Here's how the part is built. I have some questions about the finished solid (model axes, mm). A direction names the side the tool comes from. Round coordinates to 2 decimals unless told otherwise and drop trailing zeros. Order: outer loops, then holes, each group sorted by start corner. A loop starts at its lowest first (then second) coordinate and runs counter-clockwise, first axis right, second up. Notation, with made-up numbers: (-11, 47) - (31, 47) arc R24 cw to (31, 69) - close; hole circle Ø10 at (24, -27.5). An arc over 180 degrees is marked (long way). One line per item, written item: value.
from build123d import *

# Parameters (mm, degrees)
BOSS_EXTRUDE1_DEPTH = 60
FILLET2_R           = 5
SKETCH5_R           = 5.5
CUT_EXTRUDE1_DEPTH  = 105.256230261


with BuildPart() as part:
    # Sketch2 → Boss-Extrude1 (new body)
    with BuildSketch(Plane.XY):
        with BuildLine():
            Line((-26, 45.665759035), (-26, 5.665759035))
            ThreePointArc((-26, 5.665759035), (0, -15.794380862), (26, 5.665759035))
            Line((26, 5.665759035), (26, 45.665759035))
            Line((26, 45.665759035), (36, 45.665759035))
            Line((36, 45.665759035), (36, 2.642754473))
            Line((36, 2.642754473), (36, -34.334240965))
            Line((36, -34.334240965), (-36, -34.334240965))
            Line((-36, -34.334240965), (-36, 5.665759035))
            Line((-36, 5.665759035), (-36, 45.665759035))
            Line((-36, 45.665759035), (-26, 45.665759035))
        make_face()
    extrude(amount=BOSS_EXTRUDE1_DEPTH)

    # Fillet2
    fillet2_edges = [part.edges().sort_by_distance(p)[0] for p in [
        (36, 45.665759035, 30),
        (26, 45.665759035, 30),
        (-26, 45.665759035, 30),
        (-36, 45.665759035, 30),
    ]]
    fillet(fillet2_edges, radius=FILLET2_R - 0.0001)  # a hair under: the kernel refuses the full size

    # Sketch5 → Cut-Extrude1 (cut, through all)
    with BuildSketch(Plane(origin=(36, 0, 0), x_dir=(0, 0, -1), z_dir=(1, 0, 0))):
        with Locations(Location((-30, -25.064310913, 0), (0, 0, 90))):
            Circle(SKETCH5_R)
    extrude(amount=-CUT_EXTRUDE1_DEPTH, mode=Mode.SUBTRACT)


solid = part.part
Q1. If we section it at C-C, the plane x = -9: Please give me the cut outline in (y, z), then the cut area to 3 significant figures.
Results list:
outline: (-34.33, 0) - (-14.22, 0) - (-14.22, 60) - (-34.33, 60) - close; hole circle Ø11 at (-25.06, 30)
area: 1,110 mm²
Q2. If I drill on line 1 along X through (y, z) = (10.5, 51.5); line 2 along Z through (x, y) = (-20.5, -20.5); line 3 along Z through (x, y) = (17, -23.5), over which ranges is the centre line in solid material (lowest first)?
Results list:
line 1: -36 to -26, 26 to 36
line 2: 0 to 26.93, 33.07 to 60
line 3: 0 to 24.73, 35.27 to 60
Q3. If we section it at A-A, the plane y = 25.5: Please give me the cut outline in (x, z).
Results list:
outline: (-36, 0) - (-26, 0) - (-26, 60) - (-36, 60) - close; (26, 0) - (36, 0) - (36, 60) - (26, 60) - close
Q4. We'd pull the mould along X, two halves only. Please class faces 3 (the flat face through (1, -20, 0)), 4 (the cylindrical face through (27.426, 44.162, 30.42)), 5 (the cylindrical face through (34.496, 44.24, 30.42)): released by +X, released by -X, zero draft, split by the parting line, or undercut.
Results list:
face 3: zero draft
face 4: undercut
face 5: released by +X
Q5. Which directions (+Z, -Z, +X, -X, +Y, -Y) give clear straight access to the entire face, cutting with the end or side of a thin tool? Please do faces 1 (the cylindrical face through (-27.426, 44.162, 30.42)), 2 (the cylindrical face through (0.504, -25.78, 35.453)).
Results list:
face 1: +Z, -Z, +Y
face 2: +X, -X
Q6. Will these pins go through, and if not, where does the flat tip stop? pin 1 (12 mm diameter, centred on x = -6.5, z = 35.5, fed in from +Y); pin 2 (8 mm diameter, centred on x = 18.5, y = 18, fed in from +Z) (1 decimal).
Results list:
pin 1: y = -12.66
pin 2: through
